Geometry check sheet. Reference: the model listing, model coordinates, mm. A direction names the side the tool comes from. Coordinates: 2 decimals unless noted, no trailing zeros. Write each loop counter-clockwise with the first axis right and the second up, starting at its lowest first coordinate (ties: lowest second). Pieces come first, ordered by that corner, then holes. Notation, with made-up numbers: (13, -25.5) -> (40, -25.5) arc R26 ccw to (40, 8.5) -> close; hole circle Ø11 at (84.25, 21.5). An arc over 180 degrees is marked (long way). One line per question, with ' | ' between items.
from build123d import *

# Parameters (mm, degrees)
F1_DEPTH = 10
F2_R     = 2
F3_DEPTH = 25
F4_R     = 2
F5_DEPTH = 25


with BuildPart() as f1:
    # F0 (on Top) → F1 (new body)
    with BuildSketch(Plane.XY):
        with BuildLine():
            ThreePointArc((-0.5, -4.220485754), (-4.25, 0), (-0.5, 4.220485754))
            Line((-0.5, 4.220485754), (-0.5, 9.236476601))
            Line((-0.5, 9.236476601), (-0.5, 19.236476601))
            Line((-0.5, 19.236476601), (-4, 19.236476601))
            Line((-4, 19.236476601), (-4, 8.3404136588))
            ThreePointArc((-4, 8.3404136588), (-9.2496585868, 0.0794734394), (-4.1427212192, -8.2704510699))
            Line((-4.1427212192, -8.2704510699), (-4, -19.236476601))
            Line((-4, -19.236476601), (-0.5, -19.236476601))
            Line((-0.5, -19.236476601), (-0.5, -9.236476601))
            Line((-0.5, -9.236476601), (-0.5, -4.220485754))
        make_face()
    extrude(amount=F1_DEPTH)

    # F2 (on face) → F3 (cut)
    with BuildSketch(Plane(origin=(-4, 0, 0), x_dir=(0, -1, 0), z_dir=(-1, 0, 0))):
        with Locations((-13.7884451299, 5)):
            Circle(F2_R)
    extrude(amount=-F3_DEPTH, mode=Mode.SUBTRACT)

    # F4 (on face) → F5 (cut)
    with BuildSketch(Plane(origin=(-4.2496400996, -0.0553084447, 0), x_dir=(0.0130137517, -0.9999153175, 0), z_dir=(-0.9999153175, -0.0130137517, 0))):
        with Locations((13.6993154824, 5)):
            Circle(F4_R)
    extrude(amount=-F5_DEPTH, mode=Mode.SUBTRACT)


solid = f1.part
1. Go/stop test with flat-tipped pins: P1, Ø3.5, axis at y = 13.79, z = 5, coming from the +X side; P2, Ø5, axis at y = 13, z = 4, coming from the -X side; P3, Ø3, axis at x = -6.5, z = 6, coming from the -Y side. Record where each tip stops, or that it passes through.
Worked answers:
P1: through | P2: x = -4 | P3: y = -7.78
2. Material ranges on line 1 (X direction, y = 0, z = 3.75); line 2 (X direction, y = 8.5, z = 7.5); line 3 (Y direction, x = -3.25, z = 1), recorded low to high. Write a range as from..to.
Worked answers:
line 1: -9.25..-4.25 | line 2: -4..-0.5 | line 3: -19.24..-2.74, 2.74..19.24
3. Mould release check, pull along Y, two halves, no side actions. Record for faces 3 (the face through (-5, 0, 0)), 4 (the face through (-2.27, -15.64, 5.6)), 5 (the face through (-9.247, 0.224, 4.93)): released by +Y, released by -Y, zero draft, split by the parting line, or undercut.
Worked answers:
face 3: zero draft | face 4: undercut | face 5: split by the parting line
4. Tool access check on faces 1 (the face through (-2, 19.236, 5)), 2 (the face through (-4, 13.9, 2.7)). Record the directions out of +Z, -Z, +X, -X, +Y, -Y that give a thin tool (end or side, any length) a straight path to the whole face; none if there is none.
Worked answers:
face 1: +Z, -Z, +X, -X, +Y | face 2: +Z, -Z, -X, +Y
5. Cross-section at B-B on z = 6.5. Record the boundary of the cut face in (x, y), and give its area (3 significant figures).
Worked answers:
outline: (-4.14, -8.27) -> (-4.09, -12.43) -> (-0.5, -12.38) -> (-0.5, -4.22) arc R4.25 cw to (-0.5, 4.22) -> (-0.5, 12.47) -> (-4, 12.47) -> (-4, 8.34) arc R9.25 ccw to start; (-4.05, -15.08) -> (-4, -19.24) -> (-0.5, -19.24) -> (-0.5, -15.03) -> close; (-4, 15.11) -> (-0.5, 15.11) -> (-0.5, 19.24) -> (-4, 19.24) -> close | area: 155 mm²
6. Cross-section at A-A on y = 12.5. Record the boundary of the cut face in (x, z), and give its area (3 significant figures).
Worked answers:
outline: (-4, 0) -> (-0.5, 0) -> (-0.5, 3.47) -> (-4, 3.47) -> close; (-4, 6.53) -> (-0.5, 6.53) -> (-0.5, 10) -> (-4, 10) -> close | area: 24.3 mm²
7. Cross-section at D-D on x = -6.75. Record the boundary of the cut face in (y, z).
Worked answers:
outline: (-6.32, 0) -> (6.32, 0) -> (6.32, 10) -> (-6.32, 10) -> close
8. Cross-section at C-C on z = 1.5. Record the boundary of the cut face in (x, y).
Worked answers:
outline: (-4.14, -8.27) -> (-4, -19.24) -> (-0.5, -19.24) -> (-0.5, -4.22) arc R4.25 cw to (-0.5, 4.22) -> (-0.5, 19.24) -> (-4, 19.24) -> (-4, 8.34) arc R9.25 ccw to start
